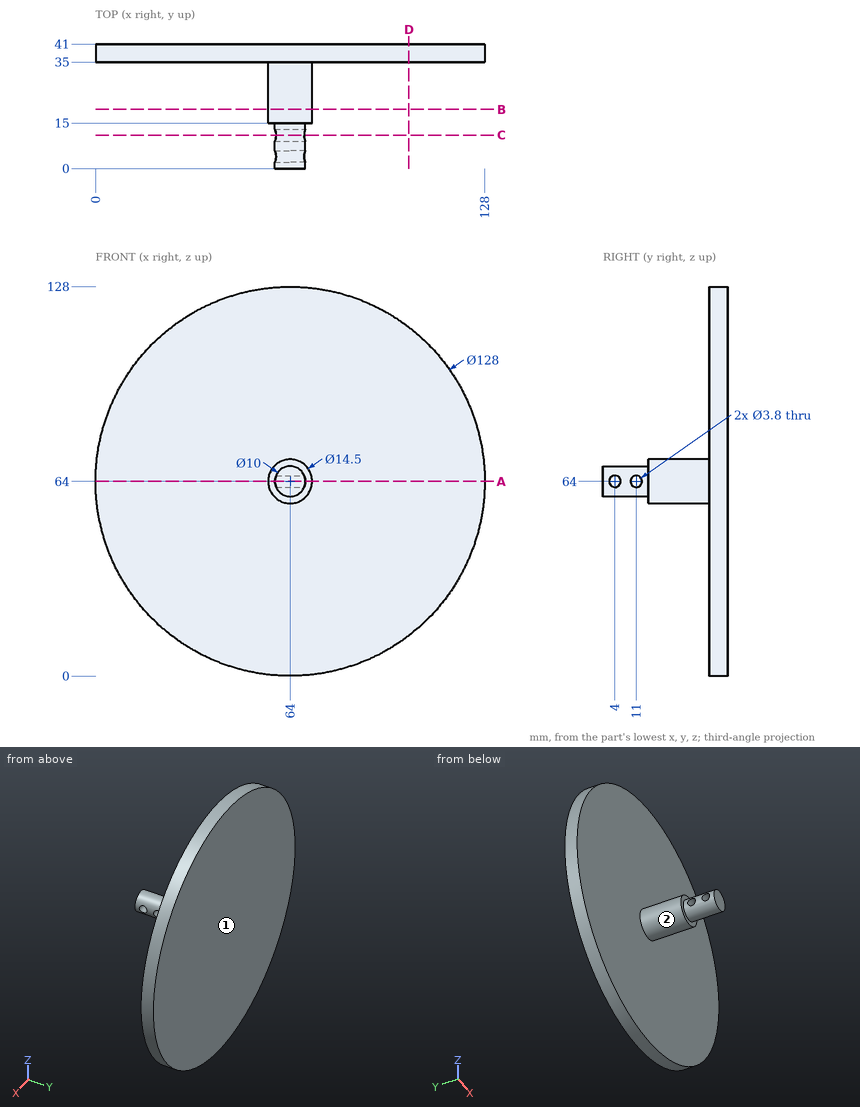
Check sheet for the drawn part. Datum: minimum x, y, z corner. Units: mm. A direction names the side the tool comes from. Give positions to 0.01 mm unless a question says otherwise; leave off trailing zeros. Write each loop counter-clockwise with the first axis right and the second up, starting at its lowest first coordinate (ties: lowest second). Pieces come first, ordered by that corner, then holes. Notation, with made-up numbers: (-38, 1) -> (-33, 1) arc R13 cw to (-33, 12) -> close; hole circle Ø3 at (10, -17.5). An arc over 180 degrees is marked (long way). Use one line per item in the form item = value. Start each with the question number.
1. Go/stop test with flat-tipped pins: P1, Ø4.5, axis at y = 11, z = 64, coming from the +X side; P2, Ø1.5, axis at x = 58.5, y = 28.5, coming from the -Z side; P3, Ø1, axis at x = 61, z = 109, coming from the -Y side. Record where each tip stops, or that it passes through.
2. Section check A-A (z = 64). Record the cut outline in (x, y), and give its area (3 significant figures).
3. Thickness scan on line 1 along Y through (x, z) = (60.1, 64); line 2 along Y through (x, z) = (78.5, 19); line 3 along X through (y, z) = (38, 111.5). Record the ranges inside material, lowest first. Write a range as from..to.
4. Access from +Z, -Z, +X, -X, +Y, -Y to the whole of each face (thin tool, end or side, straight path). Record for the marked faces 1 and 2.
5. Section check B-B (y = 19.5). Record the cut outline in (x, z), and give its area (3 significant figures).
6. Section check C-C (y = 11). Record the cut outline in (x, z), and give its area (3 significant figures).
7. Section check D-D (x = 103). Record the cut outline in (y, z).
Conclusion:
q1.P1 = 69
q1.P2 = 58.52
q1.P3 = 35
q2.outline = (0, 35) -> (56.75, 35) -> (56.75, 15) -> (59, 15) -> (59, 12.9) -> (69, 12.9) -> (69, 15) -> (71.25, 15) -> (71.25, 35) -> (128, 35) -> (128, 41) -> (0, 41) -> close; (59, 0) -> (69, 0) -> (69, 2.1) -> (59, 2.1) -> close; (59, 5.9) -> (69, 5.9) -> (69, 9.1) -> (59, 9.1) -> close
q2.area = 1,130 mm²
q3.line_1 = 0..2.1, 5.9..9.1, 12.9..41
q3.line_2 = 35..41
q3.line_3 = 21.11..106.89
q4.face_1 = +Z, -Z, +X, -X, +Y
q4.face_2 = -Y
q5.outline = circle Ø14.5 at (64, 64)
q5.area = 165 mm²
q6.outline = (59.38, 62.1) arc R5 ccw to (68.62, 62.1) -> close; (59.38, 65.9) -> (68.62, 65.9) arc R5 ccw to start
q6.area = 41.5 mm²
q7.outline = (35, 13.26) -> (41, 13.26) -> (41, 114.74) -> (35, 114.74) -> close
